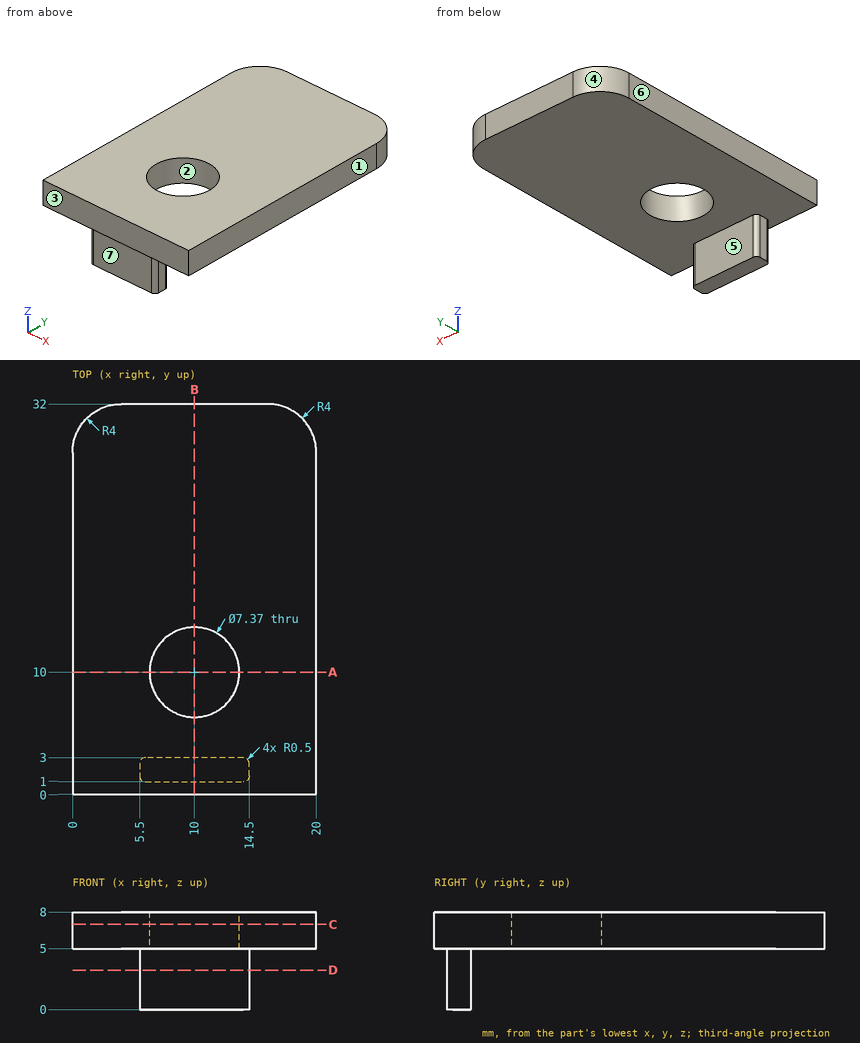
Verification items for this drawing (mm, ordinates from the low corner). A direction names the side the tool comes from. Round coordinates to 2 decimals unless told otherwise and drop trailing zeros. Write each loop counter-clockwise with the first axis right and the second up, starting at its lowest first coordinate (ties: lowest second). Pieces come first, ordered by that corner, then holes. Notation, with made-up numbers: (38.25, -32.5) - (83.25, -32.5) arc R22 cw to (83.25, -9.5) - close; hole circle Ø9 at (-22, 43). An arc over 180 degrees is marked (long way). One line per item, written item: value.
1. Cross-section at A-A on y = 10. Record the boundary of the cut face in (x, z) (3 decimals).
The answers:
outline: (0, 5) - (6.315, 5) - (6.315, 8) - (0, 8) - close; (13.685, 5) - (20, 5) - (20, 8) - (13.685, 8) - close
2. Scan lines: L1, parallel to Y at x = 10, z = 7.1 (3 decimals); L2, parallel to Z at x = 19, y = 19.5; L3, parallel to Y at x = 10, z = 0.75. Record each from-to range of solid material in increasing order.
The answers:
L1: y = 0 to 6.315, 13.685 to 32
L2: z = 5 to 8
L3: y = 1 to 3
3. Set-up check for the marked faces 5, 6 and 7: record each of +Z, -Z, +X, -X, +Y, -Y from which the full face is reachable in a straight line by a thin tool's end or side.
The answers:
face 5: -Z, +X, -X, +Y
face 6: +Z, -Z, -X, +Y, -Y
face 7: -Z, +X, -X, -Y
4. Depth check by flat-ended pin: pin 1 Ø2 at (x, y) = (6.5, 6) entering from -Z; pin 2 Ø4 at (x, z) = (12.5, 2) entering from -Y; pin 3 Ø1.1 at (y, z) = (2, 1.5) entering from -X. Enter the tip coordinate at first touch or a pass-through.
The answers:
pin 1: stops at z = 5
pin 2: stops at y = 1
pin 3: stops at x = 5.5
5. Cross-section at D-D on z = 3.25. Record the boundary of the cut face in (x, y), and give its area (3 significant figures).
The answers:
outline: (5.5, 1.5) arc R0.5 ccw to (6, 1) - (14, 1) arc R0.5 ccw to (14.5, 1.5) - (14.5, 2.5) arc R0.5 ccw to (14, 3) - (6, 3) arc R0.5 ccw to (5.5, 2.5) - close
area: 17.8 mm^2
6. Mould release check, pull along X, two halves, no side actions. Record for the marked faces 1, 2, 3 and 4: released by +X, released by -X, zero draft, split by the parting line, or undercut.
The answers:
face 1: released by +X
face 2: undercut
face 3: zero draft
face 4: released by -X
7. Cross-section at B-B on x = 10. Record the boundary of the cut face in (y, z) (3 decimals).
The answers:
outline: (0, 5) - (1, 5) - (1, 0) - (3, 0) - (3, 5) - (6.315, 5) - (6.315, 8) - (0, 8) - close; (13.685, 5) - (32, 5) - (32, 8) - (13.685, 8) - close
8. Cross-section at C-C on z = 7. Record the boundary of the cut face in (x, y) (3 decimals), and give its area (3 significant figures).
The answers:
outline: (0, 0) - (20, 0) - (20, 28) arc R4 ccw to (16, 32) - (4, 32) arc R4 ccw to (0, 28) - close; hole circle Ø7.37 at (10, 10)
area: 590 mm^2
